For this review, take the finished solid that the model builds, in its own axes (mm). A direction names the side the tool comes from. Give positions to 0.01 mm unless a question says otherwise; leave off trailing zeros. Loops run counter-clockwise (first coordinate to the right, second up) from the corner with the lowest first, then second, coordinate; pieces in that order, holes last.
```python
from build123d import *
from build123d.topology import SkipClean

# Parameters (mm, degrees)
SKETCH1_R                    = 150
BOSS_EXTRUDE1_DEPTH          = 2.5
BOSS_EXTRUDE2_DEPTH          = 6
SKETCH3_R                    = 2.9375
BOSS_EXTRUDE3_DEPTH          = 1
BOSS_EXTRUDE4_DEPTH          = 15
CHAMFER1_SIZE                = 10
SKETCH5_R                    = 140
SKETCH5_R_2                  = 135
BOSS_EXTRUDE5_DEPTH          = 7.5
CIRPATTERN1_COUNT            = 3
CHAMFER1_OF_CIRPATTERN1_SIZE = 10
SKETCH6_R                    = 6.263847164
BOSS_EXTRUDE6_DEPTH          = 5
CUT_EXTRUDE2_REACH           = 216.467
SKETCH7_W                    = 5.549678092
SKETCH7_H                    = 5.5
CIRPATTERN2_COUNT            = 3
FILLET1_R                    = 5


with BuildPart() as part:
    # Sketch1 → Boss-Extrude1 (new body)
    with BuildSketch(Plane(origin=(0, 0, 0), x_dir=(1, 0, 0), z_dir=(0, 1, 0))):
        with Locations(Location((0, 0, 0), (0, 0, 270))):
            Circle(SKETCH1_R)
        with BuildLine():
            Line((-12.499999821, 86.600423276), (-12.506397258, 124.372786524))
            ThreePointArc((-12.506397258, 124.372786524), (-108.253175473, 62.5), (-113.963191298, -51.355535527))
            Line((-113.963191298, -51.355535527), (-81.248166446, -32.474894246))
            ThreePointArc((-81.248166446, -32.474894246), (-64.174682453, -37.051270189), (-68.748166625, -54.12552903))
            Line((-68.748166625, -54.12552903), (-101.45679404, -73.017250997))
            ThreePointArc((-101.45679404, -73.017250997), (0, -125), (101.45679404, -73.017250997))
            Line((101.45679404, -73.017250997), (68.748166625, -54.12552903))
            ThreePointArc((68.748166625, -54.12552903), (64.174682453, -37.051270189), (81.248166446, -32.474894246))
            Line((81.248166446, -32.474894246), (113.963191298, -51.355535527))
            ThreePointArc((113.963191298, -51.355535527), (108.253175473, 62.5), (12.506397258, 124.372786524))
            Line((12.506397258, 124.372786524), (12.499999821, 86.600423276))
            ThreePointArc((12.499999821, 86.600423276), (0, 74.102540378), (-12.499999821, 86.600423276))
        make_face(mode=Mode.SUBTRACT)
    extrude(amount=BOSS_EXTRUDE1_DEPTH)

    # Sketch2 → Boss-Extrude2 (add)
    with BuildSketch(Plane.XZ):
        with BuildLine():
            Line((-76.041284798, 46.048019581), (-72.100762763, 43.773847901))
            ThreePointArc((-72.100762763, 43.773847901), (-76.468319115, 40.757071843), (-76.041284798, 46.048019581))
        make_face()
        with BuildLine():
            Line((77.89939715, 42.829674582), (73.959645685, 40.554168234))
            ThreePointArc((73.959645685, 40.554168234), (73.530819157, 45.844971017), (77.89939715, 42.829674582))
        make_face()
        with BuildLine():
            Line((-1.858112352, -88.877694162), (-1.858882922, -84.328016136))
            ThreePointArc((-1.858882922, -84.328016136), (2.937499958, -86.602042859), (-1.858112352, -88.877694162))
        make_face()
    extrude(amount=BOSS_EXTRUDE2_DEPTH)

    # Sketch3 → Boss-Extrude3 (add)
    with SkipClean():  # the faces are left unmerged after this step: merging them gives an invalid solid
        with BuildSketch(Plane.XZ):
            with Locations(Location((-75, 43.301270189, 0), (0, 0, 110.761573949))):
                Circle(SKETCH3_R)
            with Locations(Location((75, 43.301270189, 0), (0, 0, 350.761573949))):
                Circle(SKETCH3_R)
            with Locations(Location((0, -86.602540378, 0), (0, 0, 129.257834216))):
                Circle(SKETCH3_R)
        extrude(amount=BOSS_EXTRUDE3_DEPTH)

    # Sketch4 → Boss-Extrude4 (add)
    with SkipClean():  # the faces are left unmerged after this step: merging them gives an invalid solid
        with BuildSketch(Plane.XZ):
            Polygon((-128.89230729, 63.194244449), (-84.389895617, 37.50076509), (-82.639895617, 40.531854003), (-127.14230729, 66.225333363), align=None)
            Polygon((-120.923974711, 76.995801328), (-76.421563038, 51.302321968), (-74.671563038, 54.333410882), (-119.173974711, 80.026890241), align=None)
        boss_extrude4 = extrude(amount=BOSS_EXTRUDE4_DEPTH)

    # Chamfer1
    chamfer1_edges = [part.edges().sort_by_distance(p)[0] for p in [
        (-128.01730729, -15, 64.709788906),
        (-83.514895617, -15, 39.016309547),
        (-120.048974711, -15, 78.511345784),
        (-75.546563038, -15, 52.817866425),
    ]]
    chamfer(chamfer1_edges, length=CHAMFER1_SIZE)

    # Sketch5 → Boss-Extrude5 (add)
    with SkipClean():  # the faces are left unmerged after this step: merging them gives an invalid solid
        with BuildSketch(Plane.XZ):
            Circle(SKETCH5_R)
            Circle(SKETCH5_R_2, mode=Mode.SUBTRACT)
        extrude(amount=BOSS_EXTRUDE5_DEPTH)

    # CirPattern1: Boss-Extrude4 ×3 about axis
    with SkipClean():  # the faces are left unmerged after this step: merging them gives an invalid solid
        cirpattern1_axis = Axis((0, 0, 0), (0, 1, 0))
        for i in range(1, CIRPATTERN1_COUNT):
            add(boss_extrude4.rotate(cirpattern1_axis, i * 360 / CIRPATTERN1_COUNT))

    # Chamfer1 of CirPattern1
    chamfer1_of_cirpattern1_edges = [part.edges().sort_by_distance(p)[0] for p in [
        (120.048974711, -15, 78.511345784),
        (75.546563038, -15, 52.817866425),
        (128.01730729, -15, 64.709788906),
        (83.514895617, -15, 39.016309547),
        (7.968332579, -15, -143.22113469),
        (7.968332579, -15, -91.834175972),
        (-7.968332579, -15, -143.22113469),
        (-7.968332579, -15, -91.834175972),
    ]]
    chamfer(chamfer1_of_cirpattern1_edges, length=CHAMFER1_OF_CIRPATTERN1_SIZE)

    # Sketch6 → Boss-Extrude6 (add)
    with SkipClean():  # the faces are left unmerged after this step: merging them gives an invalid solid
        with BuildSketch(Plane.XZ):
            with BuildLine():
                Line((-74.671563038, 54.333410882), (-70.140833711, 51.717593085))
                ThreePointArc((-70.140833711, 51.717593085), (-66.583677104, 38.4421039), (-79.859166289, 34.884947293))
                Line((-79.859166289, 34.884947293), (-84.389895617, 37.50076509))
                Line((-84.389895617, 37.50076509), (-83.625725577, 38.824346425))
                ThreePointArc((-83.625725577, 38.824346425), (-83.416322896, 48.160436479), (-75.435733078, 53.009829547))
                Line((-75.435733078, 53.009829547), (-74.671563038, 54.333410882))
            make_face()
            with Locations(Location((-75, 43.301270189, 0), (0, 0, 270))):
                Circle(SKETCH6_R, mode=Mode.SUBTRACT)
        boss_extrude6 = extrude(amount=BOSS_EXTRUDE6_DEPTH)

    # Sketch7 → Cut-Extrude2 (cut, up to next)
    with BuildSketch(Plane(origin=(0.936307925, 0, 1.622367408), x_dir=(0.8661100754576421, 0, -0.4998533156744661), z_dir=(0.4998533156744661, 0, 0.8661100754576421)), mode=Mode.PRIVATE) as cut_extrude2_sk1:
        with Locations((-86.602539136, -3.75)):
            Rectangle(SKETCH7_W, SKETCH7_H)
    cut_extrude2_tool1 = extrude(cut_extrude2_sk1.sketch, amount=CUT_EXTRUDE2_REACH, mode=Mode.PRIVATE) & part.part
    cut_extrude2 = cut_extrude2_tool1.solids().sort_by_distance((-74.071024, -3.75, 44.910934))[0]
    add(cut_extrude2, mode=Mode.SUBTRACT)

    # CirPattern2: Boss-Extrude6, Cut-Extrude2 ×3 about axis
    with SkipClean():  # the faces are left unmerged after this step: merging them gives an invalid solid
        cirpattern2_axis = Axis((0, 0, 0), (0, 1, 0))
        add([boss_extrude6.rotate(cirpattern2_axis, i * 360 / CIRPATTERN2_COUNT) for i in range(1, CIRPATTERN2_COUNT)])
        add([cut_extrude2.rotate(cirpattern2_axis, i * 360 / CIRPATTERN2_COUNT) for i in range(1, CIRPATTERN2_COUNT)], mode=Mode.SUBTRACT)

    # Fillet1
    fillet1_edges = [part.edges().sort_by_distance(p)[0] for p in [
        (-12.506397258, 1.25, -124.372786524),
        (-113.963191298, 1.25, 51.355535527),
        (-101.45679404, 1.25, 73.017250997),
        (101.45679404, 1.25, 73.017250997),
        (113.963191298, 1.25, 51.355535527),
        (12.506397258, 1.25, -124.372786524),
    ]]
    fillet(fillet1_edges, radius=FILLET1_R)


solid = part.part
```
Q1. Consider section C-C on x = -34. Give the boundary of the cut face in (y, z), plus the area to 3 significant figures.
Answers:
outline: (-7.5, -135.81) - (0, -135.81) - (0, -146.1) - (2.5, -146.1) - (2.5, -120.29) - (0, -120.29) - (0, -130.65) - (-7.5, -130.65) - close; (-7.5, 130.65) - (0, 130.65) - (0, 120.29) - (2.5, 120.29) - (2.5, 146.1) - (0, 146.1) - (0, 135.81) - (-7.5, 135.81) - close
area: 206 mm2
Q2. For probe 1 along Z at (x, y) = (0, -2.8); probe 2 along Z at (x, y) = (91.5, -2.25); probe 3 along Z at (x, y) = (-75, -3.25), list the stretches that pass through material, from the lowest coordinate up.
Answers:
probe 1: z = -140 to -135, -96.32 to -92.87, -89.54 to -83.67, -80.34 to -76.88, 135 to 140
probe 2: z = -105.96 to -99.26, 41.61 to 45.65, 60.01 to 64.05, 99.26 to 105.96
probe 3: z = -118.22 to -112.25, 33.58 to 37.04, 40.36 to 45.45, 49.57 to 54.52, 112.25 to 118.22
Q3. Mouldability with a two-part tool opening along X and no side actions: class faces 1 (the cylindrical face through (66.69, -2.46, 38.26)), 2 (the flat face through (-7.99, -10.07, -138.15)) as +X half, -X half, draft (parallel to the pull), parting line (faces both ways), or undercut.
Answers:
face 1: undercut
face 2: draft
Q4. Machinability: for faces 3 (the cylindrical face through (0, -4, -135)), 4 (the cylindrical face through (-107.456, 1.232, -63.86)), 5 (the flat face through (105, -15, 52)), which of the approach directions +Z, -Z, +X, -X, +Y, -Y give a long, thin tool a straight path to every point of the face, cutting with its end or side? Answer none if there is none.
Answers:
face 3: -Y
face 4: +Y, -Y
face 5: +Z, -Z, +X, -X, -Y
Q5. Consider section D-D on z = -111. Give the boundary of the cut face in (x, y), plus the area to 3 significant figures.
Answers:
outline: (-100.89, 0) - (-85.32, 0) - (-85.32, -7.5) - (-76.84, -7.5) - (-76.84, 0) - (-57.48, 0) - (-57.48, 2.5) - (-100.89, 2.5) - close; (-12.5, 0) - (-9.72, 0) - (-9.72, -15) - (-6.22, -15) - (-6.22, 0) - (6.22, 0) - (6.22, -15) - (9.72, -15) - (9.72, 0) - (12.5, 0) - (12.5, 2.5) - (-12.5, 2.5) - close; (57.48, 0) - (76.84, 0) - (76.84, -7.5) - (85.32, -7.5) - (85.32, 0) - (100.89, 0) - (100.89, 2.5) - (57.48, 2.5) - close
area: 512 mm2
Q6. Consider section B-B on y = -12. Give the boundary of the cut face in (x, z), plus the area to 3 significant figures.
Answers:
outline: (-122.83, 59.69) - (-90.45, 41) - (-88.7, 44.03) - (-121.08, 62.73) - close; (-114.86, 73.5) - (-82.48, 54.8) - (-80.73, 57.83) - (-113.11, 76.53) - close; (-9.72, -136.22) - (-6.22, -136.22) - (-6.22, -98.83) - (-9.72, -98.83) - close; (6.22, -136.22) - (9.72, -136.22) - (9.72, -98.83) - (6.22, -98.83) - close; (80.73, 57.83) - (82.48, 54.8) - (114.86, 73.5) - (113.11, 76.53) - close; (88.7, 44.03) - (90.45, 41) - (122.83, 59.69) - (121.08, 62.73) - close
area: 785 mm2
Q7. For pin 1 Ø14 at (x, z) = (77, 46) entering from -Y; pin 2 Ø5 at (y, z) = (-9.5, 98) entering from +X; pin 3 Ø4 at (y, z) = (-1.5, -88) entering from -X; pin 4 Ø12 at (x, z) = (111.5, 109) entering from +Y, all flat-tipped, find the tip position at first contact; note any pin that passes through.
Answers:
pin 1: stops at y = -7.87
pin 2: stops at x = 101.43
pin 3: stops at x = -122.42
pin 4: stops at y = 2.5
Q8. Consider section A-A on z = 0. Give the boundary of the cut face in (x, y), plus the area to 3 significant figures.
Answers:
outline: (-150, 0) - (-140, 0) - (-140, -7.5) - (-135, -7.5) - (-135, 0) - (-125, 0) - (-125, 2.5) - (-150, 2.5) - close; (125, 0) - (135, 0) - (135, -7.5) - (140, -7.5) - (140, 0) - (150, 0) - (150, 2.5) - (125, 2.5) - close
area: 200 mm2
